```python
from build123d import *

# Parameters (mm, degrees)
EXTRUDE_1_DEPTH     = 4
SKETCH_4_OUTSIDE_W  = 19.022
SKETCH_4_OUTSIDE_H  = 13.522
SKETCH_4_OUTSIDE_R  = 4
CUT_EXTRUDE_1_DEPTH = 2.2
CUT_EXTRUDE_2_DEPTH = 6.8


with BuildPart() as part:
    # Эскиз1 → Бобышка-Вытянуть1 (new body, symmetric)
    with BuildSketch(Plane.XY):
        Polygon((4, 0), (-4, 0), (-4, -2.2), (-6.75, -2.2), (-6.75, -8), (6.75, -8), (6.75, -2.2), (4, -2.2), align=None)
    extrude(amount=EXTRUDE_1_DEPTH, both=True)

    # Эскиз3 → Отверстие обработанное метчиком M41 (revolve, cut)
    with BuildSketch(Plane(origin=(0, 0, 0), x_dir=(0, 0, 1), z_dir=(1, 0, 0))):
        Polygon((0, 0), (0, 8), (2.15, 8), (1.65, 7.5), (1.65, 0.5), (2.15, 0), align=None)
    revolve(axis=Axis((0, 6.35, 0), (0, -1, 0)), mode=Mode.SUBTRACT)

    # Эскиз4 outside → Вырез-Вытянуть1 (cut)
    with BuildSketch(Plane(origin=(0, 0, 0), x_dir=(1, 0, 0), z_dir=(0, 1, 0))):
        Rectangle(SKETCH_4_OUTSIDE_W, SKETCH_4_OUTSIDE_H)
        with Locations(Location((0, 0, 0), (0, 0, 270))):  # turned: the seam where the file's is
            Circle(SKETCH_4_OUTSIDE_R, mode=Mode.SUBTRACT)
    extrude(amount=-CUT_EXTRUDE_1_DEPTH, mode=Mode.SUBTRACT)

    # Эскиз5 → Вырез-Вытянуть2 (cut, through all)
    with BuildSketch(Plane(origin=(0, -2.2, 0), x_dir=(1, 0, 0), z_dir=(0, 1, 0))):
        with BuildLine():
            Line((-6.75, 0), (-6.75, 4))
            Line((-6.75, 4), (-5.437140793, 4))
            ThreePointArc((-5.437140793, 4), (-6.413392252, 2.104970267), (-6.75, 0))
        make_face()
        with BuildLine():
            Line((6.75, 0), (6.75, -4))
            Line((6.75, -4), (5.437140793, -4))
            ThreePointArc((5.437140793, -4), (6.413392252, -2.104970267), (6.75, 0))
        make_face()
    extrude(amount=-CUT_EXTRUDE_2_DEPTH, mode=Mode.SUBTRACT)

    # Вырез-По траектории1: sweep along a path in Эскиз7
    with BuildLine(Plane.XZ.offset(8)) as sweep_1_path:
        Line((0, 6.75), (-6.75, 6.75))
        Line((-6.75, 6.75), (-6.75, 0))
        ThreePointArc((-6.75, 0), (-4.772970773, -4.772970773), (0, -6.75))
        Line((0, -6.75), (6.75, -6.75))
        Line((6.75, -6.75), (6.75, 0))
        ThreePointArc((6.75, 0), (4.772970773, 4.772970773), (0, 6.75))
    # Эскиз6 → Вырез-По траектории1 (sweep, cut)
    with BuildSketch(Plane.XY.offset(4)):
        Polygon((-6.75, -4.7), (-6.75, -8), (-4, -8), align=None)
    sweep(path=sweep_1_path.line, transition=Transition.RIGHT, mode=Mode.SUBTRACT)


solid = part.part
```
Read the model definition and answer for the solid it produces. Units are mm, in the model's axes. A direction names the side the tool comes from. Coordinates: 2 decimals unless noted, no trailing zeros. Loops run counter-clockwise (first coordinate to the right, second up) from the corner with the lowest first, then second, coordinate; pieces in that order, holes last. Notation, with made-up numbers: (3.25, 76) - (46.25, 76) arc R18 cw to (46.25, 107) - close; hole circle Ø4 at (41, 34). An arc over 180 degrees is marked (long way). Answer in a Markdown table with one row per item.
1. Find section A-A, the plane y = -3. Write down the section's boundary in (x, z).
Conclusion:
| item | result |
|---|---|
| outline | (-6.75, 0) arc R6.75 ccw to (-5.44, -4) - (6.75, -4) - (6.75, 0) arc R6.75 ccw to (5.44, 4) - (-6.75, 4) - close; hole circle Ø3.3 at (0, 0) |
2. Determine the mould class of faces 1 (the face through (-1, -4, 4)), 2 (the face through (5.36, -6.37, -1.97)), 3 (the face through (-1.115, -3.951, -1.216)), 4 (the face through (-6.75, -3, 2)) for opening direction X: +X half, -X half, draft (parallel to the pull), parting line (faces both ways), or undercut.
Conclusion:
| item | result |
|---|---|
| face 1 | draft |
| face 2 | +X half |
| face 3 | undercut |
| face 4 | -X half |
3. Which of the six approach directions +Z, -Z, +X, -X, +Y, -Y give full straight-line access (tool end or side, diameter ignored) to faces 5 (the face through (-2, 0, -2)), 6 (the face through (-3.905, -1.085, -0.867))?
Conclusion:
| item | result |
|---|---|
| face 5 | +Z, -Z, +X, -X, +Y |
| face 6 | +Y |
4. Find section C-C, the plane y = -1. Write down the section's boundary in (x, z).
Conclusion:
| item | result |
|---|---|
| outline | circle Ø8 at (0, 0); hole circle Ø3.3 at (0, 0) |
5. Find section B-B, the plane y = -5.5. Write down the section's boundary in (x, z).
Conclusion:
| item | result |
|---|---|
| outline | (-6.08, 0) arc R6.08 ccw to (-4.58, -4) - (6.08, -4) - (6.08, 0) arc R6.08 ccw to (4.58, 4) - (-6.08, 4) - close; hole circle Ø3.3 at (0, 0) |
6. Straight lines are drawn through the part: line 1 (X direction, y = -2.5, z = 0); line 2 (X direction, y = -5, z = 0); line 3 (Z direction, x = -1, y = -2.75). For each, find the intervals that lie inside material, in ascending order.
Conclusion:
| item | result |
|---|---|
| line 1 | x = -6.75 to -1.65, 1.65 to 6.75 |
| line 2 | x = -6.5 to -1.65, 1.65 to 6.5 |
| line 3 | z = -4 to -1.31, 1.31 to 4 |
